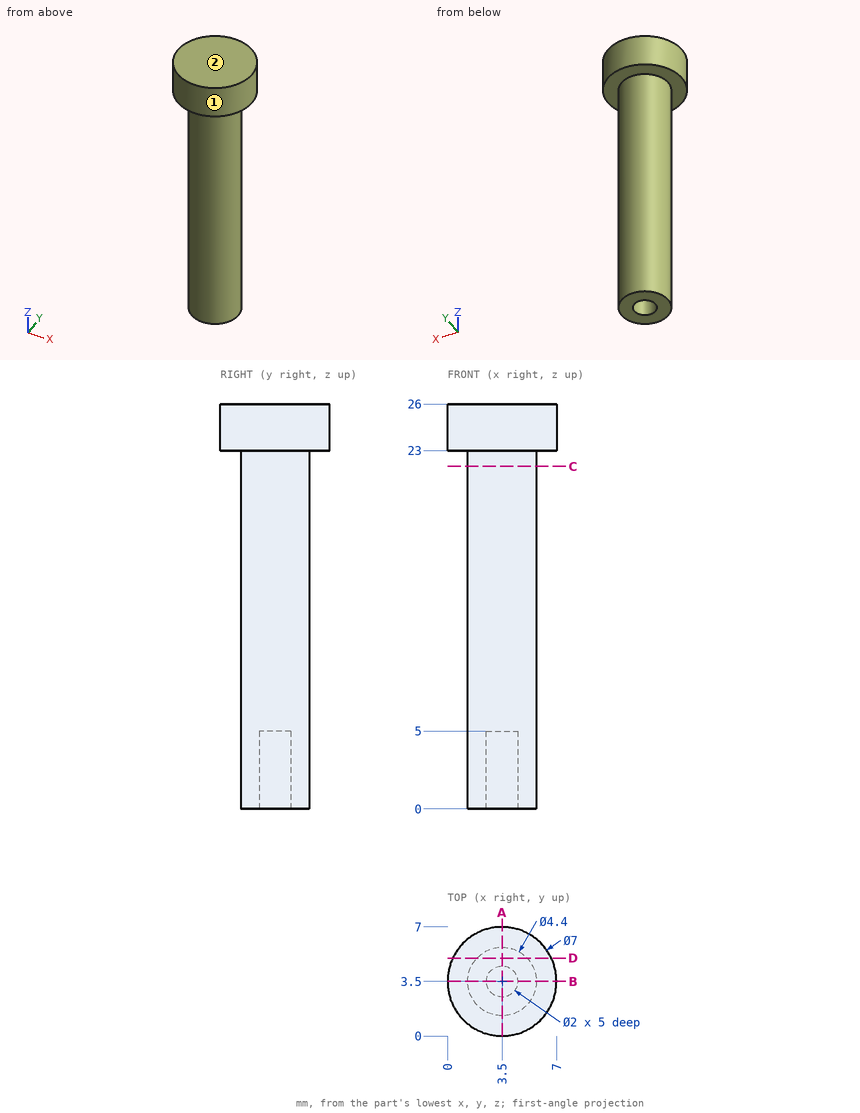
Here's the drawing with two shaded views (mm, measured from the low corner). I have some questions. Give positions to 0.01 mm unless a question says otherwise; leave off trailing zeros. Write each loop counter-clockwise with the first axis right and the second up, starting at its lowest first coordinate (ties: lowest second). Pieces come first, ordered by that corner, then holes. Notation, with made-up numbers: (81.25, 64) - (90.25, 64) arc R13 cw to (90.25, 87) - close; hole circle Ø4 at (22.5, 24). An arc over 180 degrees is marked (long way). Write item = value, one per line. Start each with the question number.
1. Thinking about a two-plate mould opening in Y: for the marked faces 1 and 2, which applies, released by +Y, released by -Y, zero draft, split by the parting line, or undercut?
2. Imagine slicing it at A-A (x = 3.5). Please give me the cut outline in (y, z).
3. Imagine slicing it at D-D (y = 5). Please give me the cut outline in (x, z), and give its area (3 significant figures).
4. Imagine slicing it at C-C (z = 22). Please give me the cut outline in (x, y).
5. Please list where these lines run through material, in increasing order: line 1 (Y direction, x = 3.5, z = 1.65); line 2 (Z direction, x = 5.5, y = 4.5); line 3 (Y direction, x = 5, z = 2.25).
6. For pin 1 (3 mm diameter, centred on y = 1, z = 8, fed in from -X); pin 2 (0.6 mm diameter, centred on x = 3.5, y = 3, fed in from -Z); pin 3 (1.5 mm diameter, centred on x = 1, y = 1, fed in from -Z), each with a flat end and sliding along its axis, tell me the tip position at first contact or that it passes through.
Worked answers:
q1.face_1 = split by the parting line
q1.face_2 = zero draft
q2.outline = (0, 23) - (1.3, 23) - (1.3, 0) - (2.5, 0) - (2.5, 5) - (4.5, 5) - (4.5, 0) - (5.7, 0) - (5.7, 23) - (7, 23) - (7, 26) - (0, 26) - close
q3.outline = (0.34, 23) - (1.89, 23) - (1.89, 0) - (5.11, 0) - (5.11, 23) - (6.66, 23) - (6.66, 26) - (0.34, 26) - close
q3.area = 93.0 mm2
q4.outline = circle Ø4.4 at (3.5, 3.5)
q5.line_1 = 1.3 to 2.5, 4.5 to 5.7
q5.line_2 = 23 to 26
q5.line_3 = 1.89 to 5.11
q6.pin_1 = 1.54
q6.pin_2 = 5
q6.pin_3 = 23
